Work out the finished part from the listing and answer in its coordinate system (mm). A direction names the side the tool comes from. Give positions to 0.01 mm unless a question says otherwise; leave off trailing zeros. Order: outer loops, then holes, each group sorted by start corner. A loop starts at its lowest first (then second) coordinate and runs counter-clockwise, first axis right, second up.
```python
from build123d import *

# Parameters (mm, degrees)
SKETCH1_R           = 100
BOSS_EXTRUDE1_DEPTH = 40
CIRPATTERN1_COUNT   = 6


with BuildPart() as part:
    # Sketch1 → Boss-Extrude1 (new body)
    with BuildSketch(Plane(origin=(0, 0, 0), x_dir=(1, 0, 0), z_dir=(0, 1, 0))):
        with Locations(Location((0, 0, 0), (0, 0, 270))):
            Circle(SKETCH1_R)
    extrude(amount=BOSS_EXTRUDE1_DEPTH)

    # Sketch2 → 1/4-20 Tapped Hole1 (revolve, cut)
    with BuildSketch(Plane(origin=(0, 40, -85), x_dir=(0, 0, 1), z_dir=(1, 0, 0))):
        Polygon((0, 0), (0, 18.043816902), (2.5527, 16.51), (2.5527, 0), align=None)
    f_1_4_20_tapped_hole1 = revolve(axis=Axis((0, 46.35, -85), (0, -1, 0)), mode=Mode.SUBTRACT)

    # CirPattern1: 1/4-20 Tapped Hole1 ×6 about axis
    cirpattern1_axis = Axis((0, 0, 0), (0, 1, 0))
    for i in range(1, CIRPATTERN1_COUNT):
        add(f_1_4_20_tapped_hole1.rotate(cirpattern1_axis, i * 360 / CIRPATTERN1_COUNT), mode=Mode.SUBTRACT)


solid = part.part
```
1. Straight lines are drawn through the part: probe 1 along X at (y, z) = (29.25, 42.5); probe 2 along Z at (x, y) = (-0.5, 20); probe 3 along X at (y, z) = (18.5, 29.5). For each, find the intervals that lie inside material, in ascending order.
Findings below:
probe 1: x = -90.52 to -76.16, -71.06 to 71.06, 76.16 to 90.52
probe 2: z = -100 to 100
probe 3: x = -95.55 to 95.55
2. The part is cut by section B-B (x = -30.5). Write down the section's boundary in (y, z), then the cut area to 3 significant figures.
Findings below:
outline: (0, -95.24) - (40, -95.24) - (40, 95.24) - (0, 95.24) - close
area: 7,620 mm2
3. Given P1, Ø1, axis at x = -46.5, y = 22.5, coming from the -Z side; P2, Ø1, axis at y = 28.5, z = -72, coming from the -X side; P3, Ø1.5, axis at x = -30.5, y = 17, coming from the +Z side, each flat-ended and moving along its own axis, determine where each tip first touches the part or whether it passes through.
Findings below:
P1: stops at z = -88.79
P2: stops at x = -69.91
P3: stops at z = 95.47
4. The part is cut by section A-A (y = 28). Write down the section's boundary in (x, z), then the cut area to 3 significant figures.
Findings below:
outline: circle Ø200 at (0, 0); hole circle Ø5.11 at (-73.61, -42.5); hole circle Ø5.11 at (-73.61, 42.5); hole circle Ø5.11 at (0, -85); hole circle Ø5.11 at (0, 85); hole circle Ø5.11 at (73.61, -42.5); hole circle Ø5.11 at (73.61, 42.5)
area: 31,300 mm2
5. The mould has two halves that part along Z. Classify faces 3 (the face through (75.877, 31.861, 43.678)), 4 (the face through (30.04, 19.72, 95.38)), 5 (the face through (-75.877, 31.861, -43.678)), 6 (the face through (1, 0, -1)): pulls with the +Z half, pulls with the -Z half, needs draft (parallel to the pull), parting line crosses it, or undercut.
Findings below:
face 3: undercut
face 4: parting line crosses it
face 5: undercut
face 6: needs draft
6. Which of the six approach directions +Z, -Z, +X, -X, +Y, -Y give full straight-line access (tool end or side, diameter ignored) to faces 1 (the face through (1, 40, -1)), 2 (the face through (73.72, 31.86, -39.95))?
Findings below:
face 1: +Z, -Z, +X, -X, +Y
face 2: +Y
7. The part is cut by section C-C (z = 55). Write down the section's boundary in (x, y), then the cut area to 3 significant figures.
Findings below:
outline: (-83.52, 0) - (83.52, 0) - (83.52, 40) - (-83.52, 40) - close
area: 6,680 mm2
